For this review, take the finished solid that the model builds, in its own axes (mm). Face numbers are marked on the shaded views. A direction names the side the tool comes from. Give positions to 0.01 mm unless a question says otherwise; leave off trailing zeros. Write each loop counter-clockwise with the first axis right and the second up, starting at its lowest first coordinate (ties: lowest second). Pieces come first, ordered by that corner, then holes.
1) We need section A-A on x = 362.5. Give the boundary of the cut face in (y, z), and give its area (3 significant figures).
2) Draft analysis for pull direction Y (two halves, no side actions). For the marked faces 3, 4, 5 and 6, state which applies: pulls with the +Y half, pulls with the -Y half, needs draft (parallel to the pull), parting line crosses it, or undercut.
3) Machinability: for the marked faces 1 and 2, which of the approach directions +Z, -Z, +X, -X, +Y, -Y give a long, thin tool a straight path to every point of the face, cutting with its end or side? Answer none if there is none.
4) We need section B-B on z = 12.5. Give the boundary of the cut face in (x, y).
5) Wall thickness on line 1 along Y through (x, z) = (409.5, 6); line 2 along X through (y, z) = (387, 34); line 3 along X through (y, z) = (344, 56): over which ranges is each line inside the solid? List them lowest first.
6) We need section C-C on y = 376.5. Give the boundary of the cut face in (x, z), and give its area (3 significant figures).
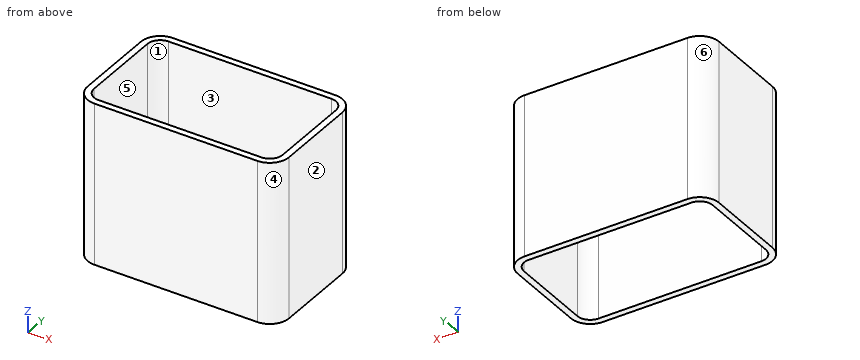
Autodesk Fusion 360 part; units mm, degrees
sketch "スケッチ1" plane through (0, 0, 0) normal (0, 0, 1) x (1, 0, 0)
  line L0 (347.8927, 333.8164) -> (448.8927, 333.8164)
  line L1 (347.8927, 337.8164) -> (448.8927, 337.8164)
  line L2 (448.8927, 408.8164) -> (347.8927, 408.8164)
  line L3 (448.8927, 404.8164) -> (347.8927, 404.8164)
  line L4 (335.8927, 396.8164) -> (335.8927, 345.8164)
  line L5 (339.8927, 396.8164) -> (339.8927, 345.8164)
  arc A0 (335.8927, 345.8164) -> (347.8927, 333.8164) centre (347.8927, 345.8164) ccw
  arc A1 (339.8927, 345.8164) -> (347.8927, 337.8164) centre (347.8927, 345.8164) ccw
  arc A2 (347.8927, 408.8164) -> (335.8927, 396.8164) centre (347.8927, 396.8164) ccw
  arc A3 (347.8927, 404.8164) -> (339.8927, 396.8164) centre (347.8927, 396.8164) ccw
  line L6 (460.8927, 345.8164) -> (460.8927, 396.8164)
  line L7 (456.8927, 345.8164) -> (456.8927, 396.8164)
  arc A4 (448.8927, 333.8164) -> (460.8927, 345.8164) centre (448.8927, 345.8164) ccw
  arc A5 (448.8927, 337.8164) -> (456.8927, 345.8164) centre (448.8927, 345.8164) ccw
  arc A6 (460.8927, 396.8164) -> (448.8927, 408.8164) centre (448.8927, 396.8164) ccw
  arc A7 (456.8927, 396.8164) -> (448.8927, 404.8164) centre (448.8927, 396.8164) ccw
  point P0 (398.3927, 371.3164)
extrude "押し出し1" add sketch "スケッチ1" along normal blind 100
Results list:
1. outline: (333.82, 0) - (337.82, 0) - (337.82, 100) - (333.82, 100) - close; (404.82, 0) - (408.82, 0) - (408.82, 100) - (404.82, 100) - close
1. area: 800 mm2
2. face 3: undercut
2. face 4: pulls with the -Y half
2. face 5: undercut
2. face 6: pulls with the +Y half
3. face 1: +Z, -Z
3. face 2: +Z, -Z, +X, +Y, -Y
4. outline: (335.89, 345.82) arc R12 ccw to (347.89, 333.82) - (448.89, 333.82) arc R12 ccw to (460.89, 345.82) - (460.89, 396.82) arc R12 ccw to (448.89, 408.82) - (347.89, 408.82) arc R12 ccw to (335.89, 396.82) - close; hole (339.89, 345.82) arc R8 ccw to (347.89, 337.82) - (448.89, 337.82) arc R8 ccw to (456.89, 345.82) - (456.89, 396.82) arc R8 ccw to (448.89, 404.82) - (347.89, 404.82) arc R8 ccw to (339.89, 396.82) - close
5. line 1: y = 333.82 to 337.82, 404.82 to 408.82
5. line 2: x = 335.89 to 339.89, 456.89 to 460.89
5. line 3: x = 336.03 to 340.1, 456.68 to 460.75
6. outline: (335.89, 0) - (339.89, 0) - (339.89, 100) - (335.89, 100) - close; (456.89, 0) - (460.89, 0) - (460.89, 100) - (456.89, 100) - close
6. area: 800 mm2
